The listing builds one solid part. Answer for the finished solid, in the listing's coordinates (mm). A direction names the side the tool comes from. Round coordinates to 2 decimals unless told otherwise and drop trailing zeros. Write each loop counter-clockwise with the first axis right and the second up, starting at its lowest first coordinate (ties: lowest second). Pieces come first, ordered by that corner, then holes.
(1) For faces 5 (the face through (3.51, 37.85, 1.48)), 6 (the face through (4.76, -11.56, 1.52)), determine the directions among +Z, -Z, +X, -X, +Y, -Y from which every point of the face is accessible in a straight line to the end or side of a thin tool.
(2) A cutting plane is placed at A-A, the plane y = 0. Give the vertices of the cut face in (x, z), and give its area (3 significant figures).
(3) The mould has two halves that part along Y. Classify faces 1 (the face through (-26.27, 26.76, 1.48)), 2 (the face through (-13.86, 18.1, 1.52)), 3 (the face through (0, -41.292, 1)), 4 (the face through (-41.292, 0, 1)): +Y half, -Y half, draft (parallel to the pull), parting line (faces both ways), or undercut.
(4) Find the intervals of material crossed by probe 1 along Y at (x, z) = (0, 2); probe 2 along Y at (x, z) = (-20, 1.1); probe 3 along Y at (x, z) = (-26, 0.6), in increasing order.
(5) A cutting plane is placed at C-C, the plane x = 15.5. Give the vertices of the cut face in (y, z).
(6) Each of these flat-tipped pins is pushed along its axis until it touches: pin 1 Ø0.9 at (x, z) = (20, 1) entering from -Y; pin 2 Ø3 at (x, y) = (-8.5, 0) entering from -Z; pin 3 Ø1.2 at (y, z) = (-40, 2) entering from +X; pin 4 Ø0.9 at (y, z) = (-25, 1.5) entering from +X. Where does it stop, or does it pass through?
(7) A cutting plane is placed at D-D, the plane y = 8.5. Give the vertices of the cut face in (x, z), and give its area (3 significant figures).
from build123d import *

# Parameters (mm, degrees)
SKETCH_1_R          = 1.6
EXTRUDE_1_DEPTH     = 3
SKETCH_3_R          = 4.5
SKETCH_3_R_2        = 1.25
CUT_EXTRUDE_1_DEPTH = 4
CUT_EXTRUDE_2_DEPTH = 4
FILLET_1_R          = 1


with BuildPart() as part:
    # ｽｹｯﾁ1 → ﾎﾞｽ - 押し出し1 (new body)
    with BuildSketch(Plane.XY):
        with BuildLine():
            Line((-3, -39.182266397), (-3, -41.291643997))
            Line((-3, -41.291643997), (3, -41.291643997))
            Line((3, -41.291643997), (3, -39.182266397))
            ThreePointArc((3, -39.182266397), (3.498945518, -37.860587373), (4.746835443, -37.198354174))
            ThreePointArc((4.746835443, -37.198354174), (26.516504294, -26.516504294), (37.198354174, -4.746835443))
            ThreePointArc((37.198354174, -4.746835443), (37.860587373, -3.498945518), (39.182266397, -3))
            Line((39.182266397, -3), (41.291643997, -3))
            Line((41.291643997, -3), (41.291643997, 3))
            Line((41.291643997, 3), (39.182266397, 3))
            ThreePointArc((39.182266397, 3), (37.860587373, 3.498945518), (37.198354174, 4.746835443))
            ThreePointArc((37.198354174, 4.746835443), (26.516504294, 26.516504294), (4.746835443, 37.198354174))
            ThreePointArc((4.746835443, 37.198354174), (3.498945518, 37.860587373), (3, 39.182266397))
            Line((3, 39.182266397), (3, 41.291643997))
            Line((3, 41.291643997), (-3, 41.291643997))
            Line((-3, 41.291643997), (-3, 39.182266397))
            ThreePointArc((-3, 39.182266397), (-3.498945518, 37.860587373), (-4.746835443, 37.198354174))
            ThreePointArc((-4.746835443, 37.198354174), (-26.516504294, 26.516504294), (-37.198354174, 4.746835443))
            ThreePointArc((-37.198354174, 4.746835443), (-37.860587373, 3.498945518), (-39.182266397, 3))
            Line((-39.182266397, 3), (-41.291643997, 3))
            Line((-41.291643997, 3), (-41.291643997, -3))
            Line((-41.291643997, -3), (-39.182266397, -3))
            ThreePointArc((-39.182266397, -3), (-37.860587373, -3.498945518), (-37.198354174, -4.746835443))
            ThreePointArc((-37.198354174, -4.746835443), (-26.516504294, -26.516504294), (-4.746835443, -37.198354174))
            ThreePointArc((-4.746835443, -37.198354174), (-3.498945518, -37.860587373), (-3, -39.182266397))
        make_face()
        with Locations((-38.291643997, 0)):
            Circle(SKETCH_1_R, mode=Mode.SUBTRACT)
        with Locations((0, -38.291643997)):
            Circle(SKETCH_1_R, mode=Mode.SUBTRACT)
        with Locations((0, 38.291643997)):
            Circle(SKETCH_1_R, mode=Mode.SUBTRACT)
        with Locations((38.291643997, 0)):
            Circle(SKETCH_1_R, mode=Mode.SUBTRACT)
    extrude(amount=EXTRUDE_1_DEPTH)

    # ｽｹｯﾁ3 → ｶｯﾄ - 押し出し1 (cut, through all)
    with BuildSketch(Plane.XY.offset(3)):
        Circle(SKETCH_3_R)
        with Locations((0, 8.5)):
            Circle(SKETCH_3_R_2)
        with Locations((8.5, 0)):
            Circle(SKETCH_3_R_2)
        with Locations((0, -8.5)):
            Circle(SKETCH_3_R_2)
        with Locations((-8.5, 0)):
            Circle(SKETCH_3_R_2)
    extrude(amount=-CUT_EXTRUDE_1_DEPTH, mode=Mode.SUBTRACT)

    # ｽｹｯﾁ4 → ｶｯﾄ - 押し出し2 (cut, through all)
    with BuildSketch(Plane.XY.offset(3)):
        with BuildLine():
            Line((-3, 33.365401241), (-3, 12.1346611))
            ThreePointArc((-3, 12.1346611), (-4.783542905, 11.548494156), (-6.459180807, 10.701821494))
            Line((-6.459180807, 10.701821494), (-21.471581131, 25.714221818))
            ThreePointArc((-21.471581131, 25.714221818), (-12.819894984, 30.949964339), (-3, 33.365401241))
        make_face()
        with BuildLine():
            Line((3, 33.365401241), (3, 12.1346611))
            ThreePointArc((3, 12.1346611), (4.783542905, 11.548494156), (6.459180807, 10.701821494))
            Line((6.459180807, 10.701821494), (21.471581131, 25.714221818))
            ThreePointArc((21.471581131, 25.714221818), (12.819894984, 30.949964339), (3, 33.365401241))
        make_face()
        with BuildLine():
            Line((33.365401241, 3), (12.1346611, 3))
            ThreePointArc((12.1346611, 3), (11.548494156, 4.783542905), (10.701821494, 6.459180807))
            Line((10.701821494, 6.459180807), (25.714221818, 21.471581131))
            ThreePointArc((25.714221818, 21.471581131), (30.949964339, 12.819894984), (33.365401241, 3))
        make_face()
        with BuildLine():
            Line((33.365401241, -3), (12.1346611, -3))
            ThreePointArc((12.1346611, -3), (11.548494156, -4.783542905), (10.701821494, -6.459180807))
            Line((10.701821494, -6.459180807), (25.714221818, -21.471581131))
            ThreePointArc((25.714221818, -21.471581131), (30.949964339, -12.819894984), (33.365401241, -3))
        make_face()
        with BuildLine():
            Line((3, -33.365401241), (3, -12.1346611))
            ThreePointArc((3, -12.1346611), (4.783542905, -11.548494156), (6.459180807, -10.701821494))
            Line((6.459180807, -10.701821494), (21.471581131, -25.714221818))
            ThreePointArc((21.471581131, -25.714221818), (12.819894984, -30.949964339), (3, -33.365401241))
        make_face()
        with BuildLine():
            Line((-3, -33.365401241), (-3, -12.1346611))
            ThreePointArc((-3, -12.1346611), (-4.783542905, -11.548494156), (-6.459180807, -10.701821494))
            Line((-6.459180807, -10.701821494), (-21.471581131, -25.714221818))
            ThreePointArc((-21.471581131, -25.714221818), (-12.819894984, -30.949964339), (-3, -33.365401241))
        make_face()
        with BuildLine():
            Line((-33.365401241, -3), (-12.1346611, -3))
            ThreePointArc((-12.1346611, -3), (-11.548494156, -4.783542905), (-10.701821494, -6.459180807))
            Line((-10.701821494, -6.459180807), (-25.714221818, -21.471581131))
            ThreePointArc((-25.714221818, -21.471581131), (-30.949964339, -12.819894984), (-33.365401241, -3))
        make_face()
        with BuildLine():
            Line((-33.365401241, 3), (-12.1346611, 3))
            ThreePointArc((-12.1346611, 3), (-11.548494156, 4.783542905), (-10.701821494, 6.459180807))
            Line((-10.701821494, 6.459180807), (-25.714221818, 21.471581131))
            ThreePointArc((-25.714221818, 21.471581131), (-30.949964339, 12.819894984), (-33.365401241, 3))
        make_face()
    extrude(amount=-CUT_EXTRUDE_2_DEPTH, mode=Mode.SUBTRACT)

    # ﾌｨﾚｯﾄ1
    fillet_1_edges = [part.edges().sort_by_distance(p)[0] for p in [
        (-41.291643997, -3, 1.5),
        (-41.291643997, 3, 1.5),
        (-3, 41.291643997, 1.5),
        (3, 41.291643997, 1.5),
        (41.291643997, 3, 1.5),
        (41.291643997, -3, 1.5),
        (3, -41.291643997, 1.5),
        (-3, -41.291643997, 1.5),
    ]]
    fillet(fillet_1_edges, radius=FILLET_1_R)


solid = part.part
Solutions:
1. face 5: +Z, -Z, +X, +Y
1. face 6: +Z, -Z
2. outline: (-41.29, 0) - (-39.89, 0) - (-39.89, 3) - (-41.29, 3) - close; (-36.69, 0) - (-9.75, 0) - (-9.75, 3) - (-36.69, 3) - close; (-7.25, 0) - (-4.5, 0) - (-4.5, 3) - (-7.25, 3) - close; (4.5, 0) - (7.25, 0) - (7.25, 3) - (4.5, 3) - close; (9.75, 0) - (36.69, 0) - (36.69, 3) - (9.75, 3) - close; (39.89, 0) - (41.29, 0) - (41.29, 3) - (39.89, 3) - close
2. area: 187 mm2
3. face 1: +Y half
3. face 2: undercut
3. face 3: -Y half
3. face 4: draft
4. probe 1: y = -41.29 to -39.89, -36.69 to -9.75, -7.25 to -4.5, 4.5 to 7.25, 9.75 to 36.69, 39.89 to 41.29
4. probe 2: y = -31.72 to -26.87, -24.24 to -15.76, -3 to 3, 15.76 to 24.24, 26.87 to 31.72
4. probe 3: y = -27.02 to -21.12, -3 to 3, 21.12 to 27.02
5. outline: (-34.15, 0) - (-29.7, 0) - (-29.7, 3) - (-34.15, 3) - close; (-19.74, 0) - (-11.26, 0) - (-11.26, 3) - (-19.74, 3) - close; (-3, 0) - (3, 0) - (3, 3) - (-3, 3) - close; (11.26, 0) - (19.74, 0) - (19.74, 3) - (11.26, 3) - close; (29.7, 0) - (34.15, 0) - (34.15, 3) - (29.7, 3) - close
6. pin 1: stops at y = -32
6. pin 2: stops at z = 0
6. pin 3: stops at x = 3
6. pin 4: stops at x = 28.35
7. outline: (-36.52, 0) - (-32.4, 0) - (-32.4, 3) - (-36.52, 3) - close; (-12.74, 0) - (-1.25, 0) - (-1.25, 3) - (-12.74, 3) - close; (1.25, 0) - (12.74, 0) - (12.74, 3) - (1.25, 3) - close; (32.4, 0) - (36.52, 0) - (36.52, 3) - (32.4, 3) - close
7. area: 93.7 mm2
